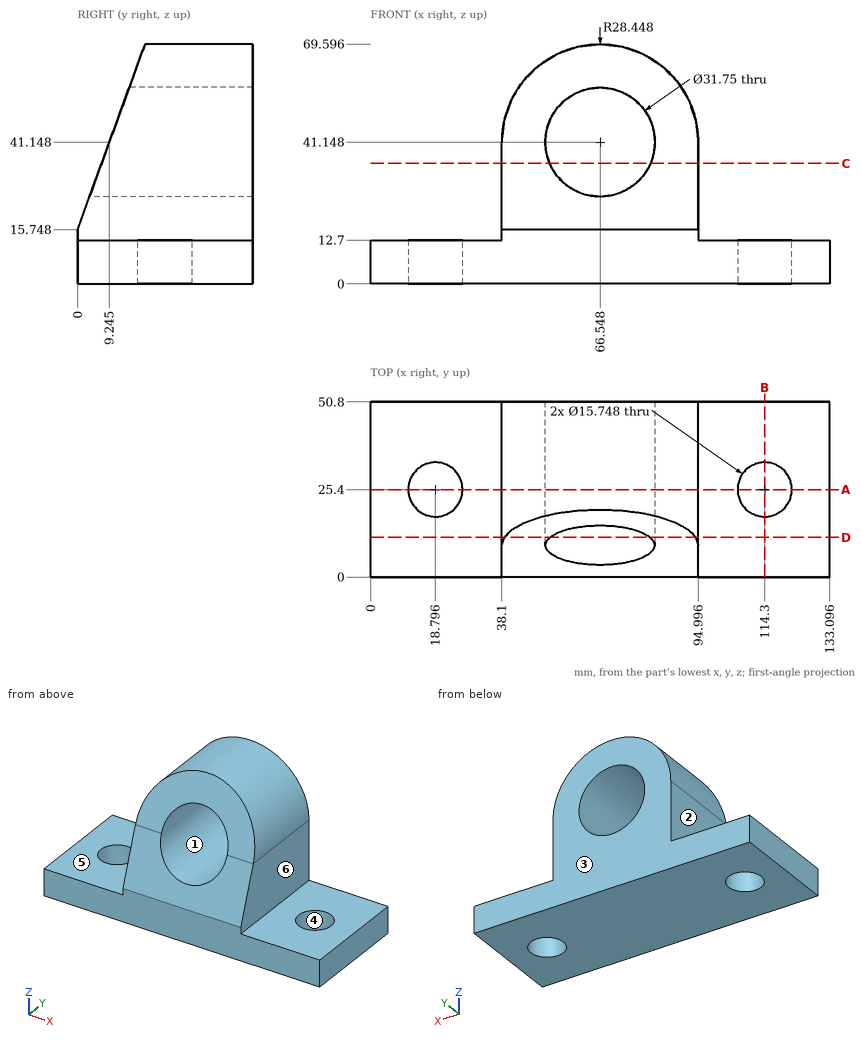
Design review of the part shown in the three views and the two pictorial views. Dimensions are in mm from the part's minimum x, y and z. A direction names the side the tool comes from. Round coordinates to 2 decimals unless told otherwise and drop trailing zeros. Loops run counter-clockwise (first coordinate to the right, second up) from the corner with the lowest first, then second, coordinate; pieces in that order, holes last. Notation, with made-up numbers: (32.25, -33) - (68.25, -33) arc R19 cw to (68.25, 2) - close; hole circle Ø4 at (85.5, -37.5). An arc over 180 degrees is marked (long way). One line per item, written item: value. Start each with the question number.
Item 1: Take a section at B-B (x = 114.3). Give the boundary of the cut face in (y, z), plus the area to 3 significant figures.
Item 2: Clearance check with flat-ended pins moving along their axes: pin 1 Ø1 at (y, z) = (27.5, 35.5) entering from -X; pin 2 Ø19 at (x, y) = (113, 26.5) entering from +Z; pin 3 Ø18 at (x, y) = (18.796, 25.4) entering from -Z; pin 4 Ø14 at (y, z) = (19.5, 24.5) entering from +X. State where each tip first meets the part, or that it passes through.
Item 3: Take a section at A-A (y = 25.4). Give the boundary of the cut face in (x, z) (3 decimals), plus the area to 3 significant figures.
Item 4: For L1, parallel to Y at x = 114, z = 7; L2, parallel to X at y = 29.5, z = 35.5; L3, parallel to Z at x = 60, y = 42, list the stretches that pass through material, from the lowest coordinate up.
Item 5: For the marked faces 4, 5 and 6, list the 3-axis set-ups (+Z, -Z, +X, -X, +Y, -Y) from which the entire face can be reached by the end or side of a thin tool; tool diameter is ignored.
Item 6: Take a section at C-C (z = 35). Give the boundary of the cut face in (x, y), plus the area to 3 significant figures.
Item 7: The part is to be moulded in two halves that separate along X. For the marked faces 1, 2 and 3, say which applies: +X half, -X half, draft (parallel to the pull), parting line (faces both ways), or undercut.
Item 8: Take a section at D-D (y = 11.5). Give the boundary of the cut face in (x, z) (3 decimals), plus the area to 3 significant figures.
Answer below:
1. outline: (0, 0) - (17.53, 0) - (17.53, 12.7) - (0, 12.7) - close; (33.27, 0) - (50.8, 0) - (50.8, 12.7) - (33.27, 12.7) - close
1. area: 445 mm2
2. pin 1: stops at x = 38.1
2. pin 2: stops at z = 12.7
2. pin 3: stops at z = 0
2. pin 4: stops at x = 95
3. outline: (0, 0) - (10.922, 0) - (10.922, 12.7) - (0, 12.7) - close; (26.67, 0) - (106.426, 0) - (106.426, 12.7) - (94.996, 12.7) - (94.996, 41.148) arc R28.448 ccw to (38.1, 41.148) - (38.1, 12.7) - (26.67, 12.7) - close; (122.174, 0) - (133.096, 0) - (133.096, 12.7) - (122.174, 12.7) - close; hole circle Ø31.75 at (66.548, 41.148)
3. area: 3,390 mm2
4. L1: y = 0 to 17.53, 33.27 to 50.8
4. L2: x = 38.1 to 51.71, 81.38 to 95
4. L3: z = 0 to 26.69, 55.61 to 68.83
5. face 4: +Z, -Z
5. face 5: +Z, -X, +Y, -Y
5. face 6: +Z, +X, +Y, -Y
6. outline: (38.1, 7.01) - (51.91, 7.01) - (51.91, 50.8) - (38.1, 50.8) - close; (81.18, 7.01) - (95, 7.01) - (95, 50.8) - (81.18, 50.8) - close
6. area: 1,210 mm2
7. face 1: undercut
7. face 2: -X half
7. face 3: draft
8. outline: (0, 0) - (133.096, 0) - (133.096, 12.7) - (94.996, 12.7) - (94.996, 41.148) arc R28.448 ccw to (94.313, 47.344) - (81.164, 47.344) arc R15.875 cw (long way) to (51.932, 47.344) - (38.783, 47.344) arc R28.448 ccw to (38.1, 41.148) - (38.1, 12.7) - (0, 12.7) - close
8. area: 3,070 mm2
